Autodesk Inventor part; units mm, degrees
ref_plane "YZ Plane" through (0, 0, 0) normal (1, 0, 0) x (0, 1, 0)
ref_plane "XZ Plane" through (0, 0, 0) normal (0, 1, 0) x (-1, 0, 0)
ref_plane "XY Plane" through (0, 0, 0) normal (0, 0, 1) x (1, 0, 0)
sketch "Sketch2" plane through (0, 0, 0) normal (0, 1, 0) x (-1, 0, 0)
  circle A0 centre (0, 0) radius 9
  circle A1 centre (0, 0) radius 8
  dimension "d91" = 18
  dimension "d92" = 16
extrude "Extrusion5" add sketch "Sketch2" along normal blind 500
sketch "Sketch3" plane through (0, 0, 0) normal (0, 0, 1) x (1, 0, 0)
  line L0 (0, 0) -> (0, 15) construction
  circle A0 centre (0, 15) radius 1.5
  line L1 (9, 500) -> (-9, 500)
  line L2 (0, 500) -> (0, 494)
  circle A1 centre (0, 494) radius 1.5
  dimension "d95" = 15
  dimension "d96" = 3
  dimension "d97" = 6
  dimension "d98" = 3
extrude "Extrusion6" cut sketch "Sketch3" along normal blind 10 and the other way blind 10
properties part number "airfoil"
Part model, mm, in its own coordinate system. Coordinates: 2 decimals unless noted, no trailing zeros. Order: outer loops, then holes, each group sorted by start corner. A loop starts at its lowest first (then second) coordinate and runs counter-clockwise, first axis right, second up. Notation, with made-up numbers: (42.5, 38.5) - (89.5, 38.5) arc R27 cw to (89.5, 72.5) - close; hole circle Ø5 at (77.5, 82). An arc over 180 degrees is marked (long way). Return JSON: item names as keys, results as strings. Group by question number.
Item 1: Drill centre lines: probe 1 along Y at (x, z) = (0, 8.7); probe 2 along X at (y, z) = (280.5, 0.75); probe 3 along X at (y, z) = (237.5, -1). Where is each one in solid material? Low to high. Write a range as from..to.
Item 2: Pin check, flat tips, straight feed: pin 1 (2.5 mm diameter, centred on x = 0, y = 15, fed in from +Z); pin 2 (1.5 mm diameter, centred on y = 244.5, z = -3.5, fed in from -X); pin 3 (1.5 mm diameter, centred on x = -1.5, y = 63.5, fed in from +Z); pin 4 (3 mm diameter, centred on y = 370.5, z = 5, fed in from -X). Stop position of each tip, or through.
Item 3: Pull direction Z, two halves, no side cores. Call faces 1 (the face through (1.172, 246.5, -8.923)), 2 (the face through (1.73, 246.5, 7.81)): pulls with the +Z half, pulls with the -Z half, needs draft (parallel to the pull), parting line crosses it, or undercut.
Item 4: Cut at B-B (y = 287). List the corners of the cut face in (x, z), plus the area to 3 significant figures.
Item 5: Cut at A-A (z = 0). List the corners of the cut face in (x, y).
Check values:
{
 "1": {"probe 1": "y = 0..13.5, 16.5..492.5, 495.5..500", "probe 2": "x = -8.97..-7.96, 7.96..8.97", "probe 3": "x = -8.94..-7.94, 7.94..8.94"},
 "2": {"pin 1": "passes through", "pin 2": "stops at x = -8.57", "pin 3": "stops at z = 8.97", "pin 4": "stops at x = -8.29"},
 "3": {"face 1": "parting line crosses it", "face 2": "undercut"},
 "4": {"outline": "circle Ø18 at (0, 0); hole circle Ø16 at (0, 0)", "area": "53.4 mm2"},
 "5": {"outline": "(-9, 0) - (-8, 0) - (-8, 500) - (-9, 500) - close; (8, 0) - (9, 0) - (9, 500) - (8, 500) - close"}
}
